from build123d import *

# Parameters (mm, degrees)
F0_W     = 25.4
F0_H     = 28.6416042886
F0_H_2   = 7.5187312844
F0_H_3   = 21.1228730042
F1_DEPTH = 71.12
F2_DEPTH = 86.36
F3_DEPTH = 17.629891634
F4_R     = 12.7
F6_D     = 10.16
F8_D     = 10.16


with BuildPart() as f1:
    # F0 (on Top) → F1 (new body)
    with BuildSketch(Plane.XY):
        with Locations((-54.5537182136, 5.834735956)):
            Rectangle(F0_W, F0_H)
        with BuildLine():
            Line((-33.6268591068, 20.1555381003), (-41.8537182136, 20.1555381003))
            Line((-41.8537182136, 20.1555381003), (-41.8537182136, -8.4860661883))
            Line((-41.8537182136, -8.4860661883), (-33.6268591068, -8.4860661883))
            Line((-33.6268591068, -8.4860661883), (-33.6268591068, -2.102764044))
            ThreePointArc((-33.6268591068, -2.102764044), (-41.5643591068, 5.834735956), (-33.6268591068, 13.772235956))
            Line((-33.6268591068, 13.772235956), (-33.6268591068, 20.1555381003))
        make_face()
        with BuildLine():
            Line((-25.4, 20.1555381003), (-33.6268591068, 20.1555381003))
            Line((-33.6268591068, 20.1555381003), (-33.6268591068, 13.772235956))
            ThreePointArc((-33.6268591068, 13.772235956), (-28.0141990311, 11.4473960317), (-25.6893591068, 5.834735956))
            ThreePointArc((-25.6893591068, 5.834735956), (-28.0141990311, 0.2220758803), (-33.6268591068, -2.102764044))
            Line((-33.6268591068, -2.102764044), (-33.6268591068, -8.4860661883))
            Line((-33.6268591068, -8.4860661883), (-25.4, -8.4860661883))
            Line((-25.4, -8.4860661883), (-25.4, 12.6368068159))
            Line((-25.4, 12.6368068159), (-25.4, 20.1555381003))
        make_face()
        with Locations((-12.7, 16.3961724581)):
            Rectangle(F0_W, F0_H_2)
        with BuildLine():
            Line((-33.6268591068, -2.102764044), (-33.6268591068, 13.772235956))
            ThreePointArc((-33.6268591068, 13.772235956), (-41.5643591068, 5.834735956), (-33.6268591068, -2.102764044))
        make_face()
        with Locations((-12.7, 2.0753703138)):
            Rectangle(F0_W, F0_H_3)
    extrude(amount=F1_DEPTH)

    # F0 (on Top) → F2 (join)
    with BuildSketch(Plane.XY):
        with BuildLine():
            Line((-33.6268591068, -2.102764044), (-33.6268591068, 13.772235956))
            ThreePointArc((-33.6268591068, 13.772235956), (-41.5643591068, 5.834735956), (-33.6268591068, -2.102764044))
        make_face()
        with BuildLine():
            ThreePointArc((-25.6893591068, 5.834735956), (-28.0141990311, 11.4473960317), (-33.6268591068, 13.772235956))
            Line((-33.6268591068, 13.772235956), (-33.6268591068, -2.102764044))
            ThreePointArc((-33.6268591068, -2.102764044), (-28.0141990311, 0.2220758803), (-25.6893591068, 5.834735956))
        make_face()
    extrude(amount=F2_DEPTH)

    # F0 (on Top) → F3 (join)
    with BuildSketch(Plane.XY):
        with BuildLine():
            ThreePointArc((-25.6893591068, 5.834735956), (-28.0141990311, 11.4473960317), (-33.6268591068, 13.772235956))
            Line((-33.6268591068, 13.772235956), (-33.6268591068, -2.102764044))
            ThreePointArc((-33.6268591068, -2.102764044), (-28.0141990311, 0.2220758803), (-25.6893591068, 5.834735956))
        make_face()
        with BuildLine():
            Line((-25.4, 20.1555381003), (-33.6268591068, 20.1555381003))
            Line((-33.6268591068, 20.1555381003), (-33.6268591068, 13.772235956))
            ThreePointArc((-33.6268591068, 13.772235956), (-28.0141990311, 11.4473960317), (-25.6893591068, 5.834735956))
            ThreePointArc((-25.6893591068, 5.834735956), (-28.0141990311, 0.2220758803), (-33.6268591068, -2.102764044))
            Line((-33.6268591068, -2.102764044), (-33.6268591068, -8.4860661883))
            Line((-33.6268591068, -8.4860661883), (-25.4, -8.4860661883))
            Line((-25.4, -8.4860661883), (-25.4, 12.6368068159))
            Line((-25.4, 12.6368068159), (-25.4, 20.1555381003))
        make_face()
        with BuildLine():
            Line((-33.6268591068, 20.1555381003), (-41.8537182136, 20.1555381003))
            Line((-41.8537182136, 20.1555381003), (-41.8537182136, -8.4860661883))
            Line((-41.8537182136, -8.4860661883), (-33.6268591068, -8.4860661883))
            Line((-33.6268591068, -8.4860661883), (-33.6268591068, -2.102764044))
            ThreePointArc((-33.6268591068, -2.102764044), (-41.5643591068, 5.834735956), (-33.6268591068, 13.772235956))
            Line((-33.6268591068, 13.772235956), (-33.6268591068, 20.1555381003))
        make_face()
        with BuildLine():
            Line((-33.6268591068, -2.102764044), (-33.6268591068, 13.772235956))
            ThreePointArc((-33.6268591068, 13.772235956), (-41.5643591068, 5.834735956), (-33.6268591068, -2.102764044))
        make_face()
    extrude(amount=-F3_DEPTH)

    # F4
    f4_edges = [f1.edges().sort_by_distance(p)[0] for p in [
        (-33.626859, -8.486066, -17.629892),
        (-33.626859, 20.155538, -17.629892),
    ]]
    fillet(f4_edges, radius=F4_R)

    # F6 (through all)
    with Locations(Plane(origin=(-41.8537182136, 0, 0), x_dir=(0, -1, 0), z_dir=(-1, 0, 0))):
        with Locations((-5.834735956, -8.814945817)):
            Hole(F6_D / 2)

    # F8 (through all)
    with Locations(Plane.YZ):
        with Locations((5.834735956, 59.3307428062)):
            Hole(F8_D / 2)


solid = f1.part
Design review of the part built by this model. Coordinates are the model's own, in mm. A direction names the side the tool comes from. Give positions to 0.01 mm unless a question says otherwise; leave off trailing zeros. Order: outer loops, then holes, each group sorted by start corner. A loop starts at its lowest first (then second) coordinate and runs counter-clockwise, first axis right, second up. Notation, with made-up numbers: (-15, 6) - (0, 6) arc R20 ccw to (0, 32) - close; hole circle Ø11 at (73, 55). An arc over 180 degrees is marked (long way). Use CSV: the item, a comma, the result in double quotes. Start each with the question number.
Q1. Take a section at C-C (z = 79). State the section outline as (x, y) points (1 decimal).
Q2. Machinability: for faces 1 (the face through (-41.854, 9.2, -4.8)), 2 (the face through (-25.4, 2, -5)), 3 (the face through (-33.512, -4.865, -13.811)), which of the approach directions +Z, -Z, +X, -X, +Y, -Y give a long, thin tool a straight path to every point of the face, cutting with its end or side? Answer none if there is none.
Q3. Take a section at D-D (y = 3). State the section outline as (x, z) points.
Q4. Take a section at A-A (x = -39.5). State the section outline as (y, z) points.
Q5. Take a section at B-B (y = 15.5). State the section outline as (x, z) points.
Q6. For P1, Ø3, axis at x = -32.5, y = -5, coming from the +Z side; P2, Ø14, axis at y = 0, z = -9.5, coming from the -X side; P3, Ø12.5, axis at x = -9.5, y = 7, coming from the -Z side, all flat-tipped, find the tip position at first contact; note any pin that passes through.
Q7. Draft analysis for pull direction Y (two halves, no side actions). For faces 4 (the face through (-33, 20.156, 33)), 5 (the face through (-34.098, 6.496, 64.368)), 6 (the face through (-13, 6, 0)), state which applies: pulls with the +Y half, pulls with the -Y half, needs draft (parallel to the pull), parting line crosses it, or undercut.
Q8. For line 1 (Z direction, x = -30.5, y = 4.25); line 2 (Z direction, x = -14, y = 15.75); line 3 (Z direction, x = -10, y = 5), list the stretches that pass through material, from the lowest coordinate up.
Calculated:
1,outline,"circle Ø15.9 at (-33.6, 5.8)"
2,face 1,"-Z, -X, +Y, -Y"
2,face 2,"-Z, +X, +Y, -Y"
2,face 3,"-Z, +X, -X, -Y"
3,outline,"(-67.25, 0) - (-41.85, 0) - (-41.85, -4.6) - (-25.4, -4.6) - (-25.4, 0) - (0, 0) - (0, 55.12) - (-67.25, 55.12) - close; (-67.25, 63.55) - (0, 63.55) - (0, 71.12) - (-26.21, 71.12) - (-26.21, 86.36) - (-41.04, 86.36) - (-41.04, 71.12) - (-67.25, 71.12) - close; (-41.85, -17.57) - (-25.4, -17.57) - (-25.4, -13.03) - (-41.85, -13.03) - close"
4,outline,"(-8.49, -4.93) arc R12.7 ccw to (4.21, -17.63) - (7.46, -17.63) arc R12.7 ccw to (20.16, -4.93) - (20.16, 71.12) - (11.17, 71.12) - (11.17, 86.36) - (0.5, 86.36) - (0.5, 71.12) - (-8.49, 71.12) - close; hole circle Ø10.16 at (5.83, -8.81); hole circle Ø10.16 at (5.83, 59.33)"
5,outline,"(-67.25, 0) - (-41.85, 0) - (-41.85, -14.76) - (-25.4, -14.76) - (-25.4, 0) - (0, 0) - (0, 71.12) - (-67.25, 71.12) - close"
6,P1,"stops at z = 71.12"
6,P2,"stops at x = -41.85"
6,P3,"stops at z = 0"
7,face 4,"pulls with the +Y half"
7,face 5,"undercut"
7,face 6,"needs draft"
8,line 1,"z = -17.63 to -13.64, -3.99 to 54.5, 64.16 to 86.36"
8,line 2,"z = 0 to 71.12"
8,line 3,"z = 0 to 54.32, 64.34 to 71.12"
